Geometry: final body of the model. Coordinates: model frame, mm. Coordinates: 2 decimals unless noted, no trailing zeros. Write each loop counter-clockwise with the first axis right and the second up, starting at its lowest first coordinate (ties: lowest second). Pieces come first, ordered by that corner, then holes. Notation, with made-up numbers: (34.5, 23.25) -> (45.5, 23.25) arc R19 cw to (45.5, 57.25) -> close; hole circle Ø2 at (46.5, 66.25). An arc over 180 degrees is marked (long way). One line per item, written item: value.
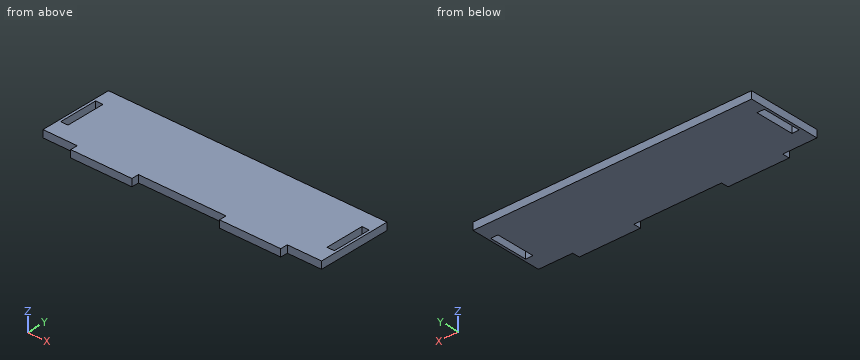
```python
from build123d import *

# Parameters (mm, degrees)
SKETCH_2_W      = 3
SKETCH_2_H      = 16
EXTRUDE_1_DEPTH = 3


with BuildPart() as part:
    # 草图2 → 凸台-拉伸1 (new body)
    with BuildSketch(Plane.XY):
        Polygon((41.5, 0), (59.4, 0), (77.3, 0), (77.3, -3), (102.3, -3), (102.3, 0), (112.3, 0), (116.3, 0), (116.3, 30), (112.3, 30), (6.5, 30), (2.5, 30), (2.5, 0), (6.5, 0), (16.5, 0), (16.5, -3), (41.5, -3), align=None)
        with Locations((5, 15)):
            Rectangle(SKETCH_2_W, SKETCH_2_H, mode=Mode.SUBTRACT)
        Polygon((112.3, 15), (112.3, 23), (115.3, 23), (115.3, 7), (112.3, 7), align=None, mode=Mode.SUBTRACT)
    extrude(amount=EXTRUDE_1_DEPTH)


solid = part.part
```
(1) Section C-C (x = 65.5). Return the cut outline in (y, z).
Responses:
outline: (0, 0) -> (30, 0) -> (30, 3) -> (0, 3) -> close
(2) Section A-A (z = 2). Return the cut outline in (x, y).
Responses:
outline: (2.5, 0) -> (16.5, 0) -> (16.5, -3) -> (41.5, -3) -> (41.5, 0) -> (77.3, 0) -> (77.3, -3) -> (102.3, -3) -> (102.3, 0) -> (116.3, 0) -> (116.3, 30) -> (2.5, 30) -> close; hole (3.5, 7) -> (6.5, 7) -> (6.5, 23) -> (3.5, 23) -> close; hole (112.3, 7) -> (115.3, 7) -> (115.3, 23) -> (112.3, 23) -> close
(3) Section B-B (y = 18). Return the cut outline in (x, z), then the cut area to 3 significant figures.
Responses:
outline: (2.5, 0) -> (3.5, 0) -> (3.5, 3) -> (2.5, 3) -> close; (6.5, 0) -> (112.3, 0) -> (112.3, 3) -> (6.5, 3) -> close; (115.3, 0) -> (116.3, 0) -> (116.3, 3) -> (115.3, 3) -> close
area: 323 mm2
(4) Line query: line 1 (X direction, y = 12.5, z = 1.7); line 2 (Y direction, x = 13, z = 0.35). Output: solid intervals per line, ascending. Write a range as [from, to].
Responses:
line 1: x = [2.5, 3.5], [6.5, 112.3], [115.3, 116.3]
line 2: y = [0, 30]
(5) First-contact query: pin 1 (5 mm diameter, centred on x = 42, y = 17, fed in from -Z); pin 2 (0.9 mm diameter, centred on y = -1.5, z = 1.5, fed in from -X); pin 3 (0.9 mm diameter, centred on x = 113.5, z = 1.5, fed in from -Y). Flat tips, straight axial feed; report the tip coordinate or a pass-through.
Responses:
pin 1: stops at z = 0
pin 2: stops at x = 16.5
pin 3: stops at y = 0
